Job drawing, mm, ordinate dimensions from the low corner. One solid piece. A direction names the side the tool comes from. Give positions to 0.01 mm unless a question says otherwise; leave off trailing zeros. Order: outer loops, then holes, each group sorted by start corner. A loop starts at its lowest first (then second) coordinate and runs counter-clockwise, first axis right, second up. Notation, with made-up numbers: M 65,-20 L 119,-20 A30 ccw 119,17 Z; hole C 71,-2.75 d9. An arc over 180 degrees is marked long. Put each result on its own line as item: value. Start each with the question number.
1) Pin check, flat tips, straight feed: pin 1 (12 mm diameter, centred on x = 180, z = 21, fed in from -Y); pin 2 (8 mm diameter, centred on y = 20, z = 150, fed in from -X); pin 3 (5 mm diameter, centred on y = 12, z = 149, fed in from +X); pin 4 (1.5 mm diameter, centred on x = 58.5, z = 130, fed in from +Y). Stop position of each tip, or through.
2) Cut at C-C (z = 75.5). Write the cut outline in (x, y), and give its area (3 significant figures).
3) Two-plate mould, pull along X, no slides. Class the marked faces 4, 5 and 6: released by +X, released by -X, zero draft, split by the parting line, or undercut.
4) Tool access for the marked faces 1, 2 and 3: list every direction of +Z, -Z, +X, -X, +Y, -Y with a clear straight run to the whole face (end or side of a thin tool).
5) Cut at A-A (y = 25). Write the cut outline in (x, z).
6) Drill centre lines: line 1 (X direction, y = 6, z = 78); line 2 (Z direction, x = 136.5, y = 21.5); line 3 (X direction, y = 5, z = 148.5). Where is each one in solid material? Low to high. Write a range as [from, to].
7) Cut at B-B (x = 34). Write the cut outline in (y, z), and give its area (3 significant figures).
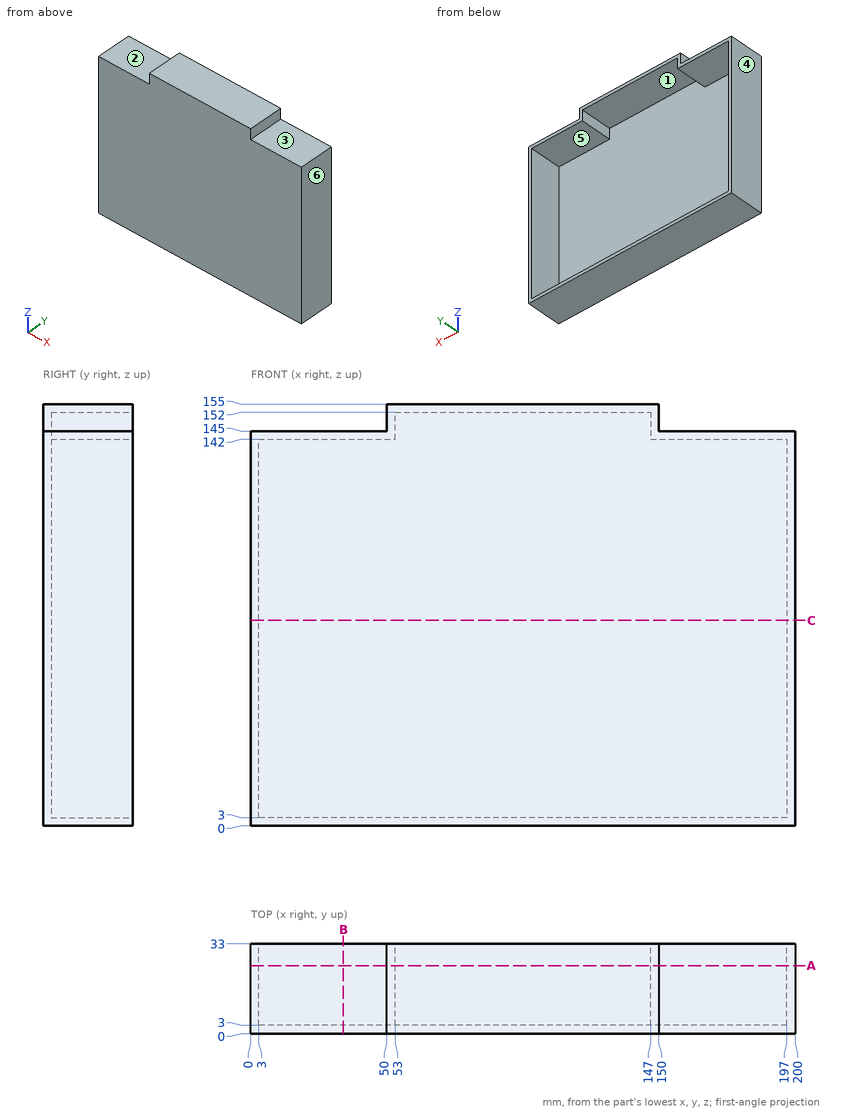
Solution:
1. pin 1: y = 0
1. pin 2: x = 50
1. pin 3: x = 150
1. pin 4: y = 3
2. outline: M 0,0 L 200,0 L 200,33 L 197,33 L 197,3 L 3,3 L 3,33 L 0,33 Z
2. area: 780 mm²
3. face 4: released by -X
3. face 5: undercut
3. face 6: released by +X
4. face 1: +Y
4. face 2: +Z, -X, +Y, -Y
4. face 3: +Z, +X, +Y, -Y
5. outline: M 0,0 L 200,0 L 200,145 L 150,145 L 150,155 L 50,155 L 50,145 L 0,145 Z; hole M 3,3 L 197,3 L 197,142 L 147,142 L 147,152 L 53,152 L 53,142 L 3,142 Z
6. line 1: [0, 3], [197, 200]
6. line 2: [0, 3], [152, 155]
6. line 3: [50, 53], [147, 150]
7. outline: M 0,0 L 33,0 L 33,3 L 3,3 L 3,142 L 33,142 L 33,145 L 0,145 Z
7. area: 615 mm²
